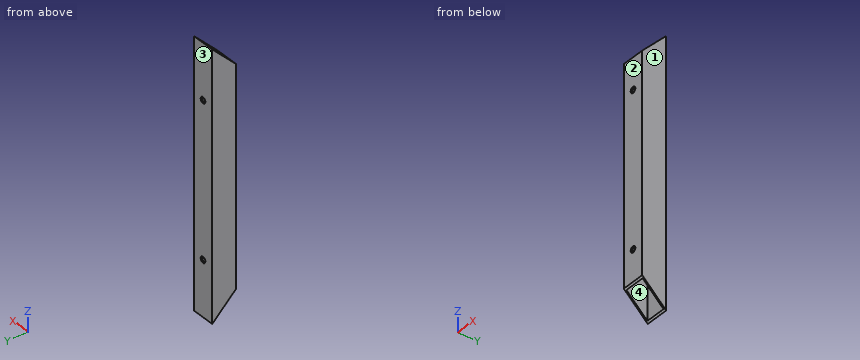
```python
from build123d import *

# Parameters (mm, degrees)
SKETCH1_W           = 50.8
SKETCH1_H           = 50.8
SKETCH1_W_2         = 44.45
SKETCH1_H_2         = 44.45
EXTRUDE_THIN1_DEPTH = 279.4
CUT_EXTRUDE1_START  = -51.8
CUT_EXTRUDE1_DEPTH  = 52.8
SKETCH3_R           = 6.35
CUT_EXTRUDE2_DEPTH  = 51.8


with BuildPart() as part:
    # Sketch1 → Extrude-Thin1 (new body)
    with BuildSketch(Plane.XY.offset(91.6)):
        with Locations((514.35, 1092.2)):
            Rectangle(SKETCH1_W, SKETCH1_H)
        with Locations((514.35, 1092.2)):
            Rectangle(SKETCH1_W_2, SKETCH1_H_2, mode=Mode.SUBTRACT)
    extrude_thin1 = extrude(amount=EXTRUDE_THIN1_DEPTH)

    # Sketch2 → Cut-Extrude1 (cut)
    with BuildSketch(Plane(origin=(539.75, 0, 0), x_dir=(0, 0, -1), z_dir=(1, 0, 0)).offset(CUT_EXTRUDE1_START)):
        Polygon((-779.680330653, 1526.280330653), (-371, 1117.6), (-320.2, 1066.8), (88.480330653, 658.119669347), (-728.880330653, -159.24099196), (-1597.04099196, 708.919669347), align=None)
    cut_extrude1 = extrude(amount=CUT_EXTRUDE1_DEPTH, mode=Mode.SUBTRACT)

    # Sketch3 → Cut-Extrude2 (cut, through all)
    with BuildSketch(Plane(origin=(0, 1117.6, 0), x_dir=(1, 0, 0), z_dir=(0, 1, 0))):
        with Locations((514.35, -254)):
            Circle(SKETCH3_R)
        with Locations((507.848069556, 254)):
            Circle(SKETCH3_R)
    cut_extrude2 = extrude(amount=-CUT_EXTRUDE2_DEPTH, mode=Mode.SUBTRACT)

    # Mirror1: Extrude-Thin1, Cut-Extrude1, Cut-Extrude2 across plane
    add(extrude_thin1.mirror(Plane(origin=(488.95, 1066.8, 91.6), x_dir=(1, 0, 0), z_dir=(0, 0, 1))))
    add(cut_extrude1.mirror(Plane(origin=(488.95, 1066.8, 91.6), x_dir=(1, 0, 0), z_dir=(0, 0, 1))), mode=Mode.SUBTRACT)
    add(cut_extrude2.mirror(Plane(origin=(488.95, 1066.8, 91.6), x_dir=(1, 0, 0), z_dir=(0, 0, 1))), mode=Mode.SUBTRACT)


solid = part.part
```
Can you work these out from the model? Positions are in its coordinate system, mm. Face numbers are marked on the shaded views. Round coordinates to 2 decimals unless told otherwise and drop trailing zeros. Loops run counter-clockwise (first coordinate to the right, second up) from the corner with the lowest first, then second, coordinate; pieces in that order, holes last. Notation, with made-up numbers: (70.25, -18) -> (77.25, -18) arc R36 cw to (77.25, 21) -> close; hole circle Ø11 at (48.5, -32). An arc over 180 degrees is marked (long way). Answer in a Markdown table with one row per item.
Item 1: We'd pull the mould along Y, two halves only. Please class the marked faces 1, 2, 3 and 4: released by +Y, released by -Y, zero draft, split by the parting line, or undercut.
Answer block:
| item | result |
|---|---|
| face 1 | zero draft |
| face 2 | released by -Y |
| face 3 | released by +Y |
| face 4 | undercut |
Item 2: If I drill on probe 1 along X at (y, z) = (1067.5, 254); probe 2 along Y at (x, z) = (507.5, -9.5) (3 decimals); probe 3 along X at (y, z) = (1077.5, 270.5) (3 decimals), over which ranges is the centre line in solid material (lowest first)?
Answer block:
| item | result |
|---|---|
| probe 1 | 488.95 to 508, 520.7 to 539.75 |
| probe 2 | 1066.8 to 1069.975, 1114.425 to 1117.6 |
| probe 3 | 488.95 to 492.125, 536.575 to 539.75 |
Item 3: Suppose I cut it at A-A, the plane y = 1104.5. List the corners of the cut face in (x, z) for me (3 decimals), plus the area to 3 significant figures.
Answer block:
| item | result |
|---|---|
| outline | (488.95, -174.7) -> (492.125, -174.7) -> (492.125, 357.9) -> (488.95, 357.9) -> close; (536.575, -174.7) -> (539.75, -174.7) -> (539.75, 357.9) -> (536.575, 357.9) -> close |
| area | 3,380 mm² |
Item 4: Suppose I cut it at B-B, the plane z = 200.5. List the corners of the cut face in (x, y) for me (3 decimals).
Answer block:
| item | result |
|---|---|
| outline | (488.95, 1066.8) -> (539.75, 1066.8) -> (539.75, 1117.6) -> (488.95, 1117.6) -> close; hole (492.125, 1069.975) -> (536.575, 1069.975) -> (536.575, 1114.425) -> (492.125, 1114.425) -> close |
Item 5: Suppose I cut it at C-C, the plane x = 497.5. List the corners of the cut face in (y, z) for me (3 decimals), plus the area to 3 significant figures.
Answer block:
| item | result |
|---|---|
| outline | (1066.8, -137) -> (1069.975, -140.175) -> (1069.975, 323.375) -> (1066.8, 320.2) -> close; (1114.425, -184.625) -> (1117.6, -187.8) -> (1117.6, 371) -> (1114.425, 367.825) -> close |
| area | 3,230 mm² |
